Geometry check sheet. Reference: drawing and pictorial views, mm from the part's lowest x, y, z. A direction names the side the tool comes from. Give positions to 0.01 mm unless a question says otherwise; leave off trailing zeros. Write each loop counter-clockwise with the first axis right and the second up, starting at its lowest first coordinate (ties: lowest second). Pieces come first, ordered by that corner, then holes. Notation, with made-up numbers: M 8.25,35 L 43.25,35 A19 cw 43.25,55 Z; hole C 48.25,20 d1. An arc over 180 degrees is marked long. Answer as a JSON object with one key per item and string values.
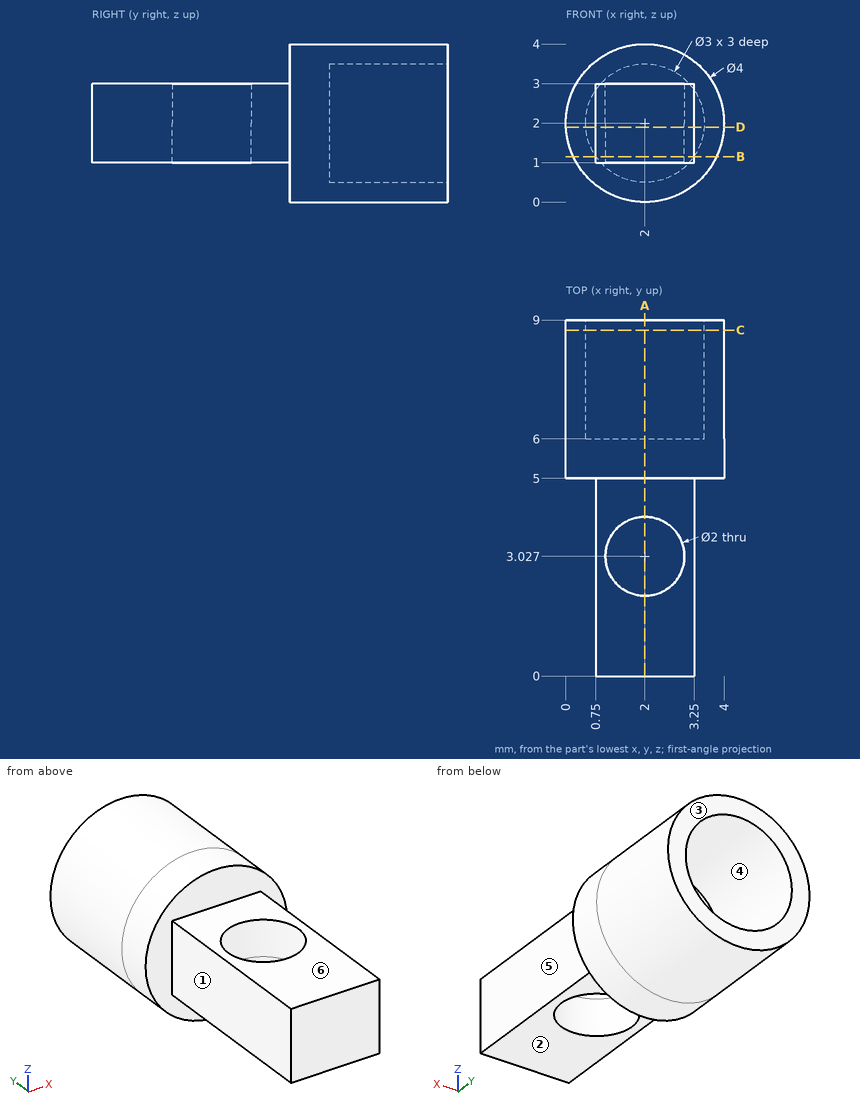
1) Section check D-D on z = 1.9. Record the boundary of the cut face in (x, y), and give its area (3 significant figures).
Completed:
{"outline": "M 0,5 L 0.75,5 L 0.75,0 L 3.25,0 L 3.25,5 L 4,5 L 4,9 L 3.5,9 L 3.5,6 L 0.5,6 L 0.5,9 L 0,9 Z; hole C 2,3.03 d2", "area": "16.4 mm2"}
2) Section check B-B on z = 1.15. Record the boundary of the cut face in (x, y).
Completed:
{"outline": "M 0.19,5 L 0.75,5 L 0.75,0 L 3.25,0 L 3.25,5 L 3.81,5 L 3.81,9 L 3.24,9 L 3.24,6 L 0.76,6 L 0.76,9 L 0.19,9 Z; hole C 2,3.03 d2"}
3) Thickness scan on L1, parallel to Y at x = 2, z = 2.6; L2, parallel to Z at x = 2, y = 6.8; L3, parallel to Y at x = 3.55, z = 1.8. Record the ranges inside material, lowest first.
Completed:
{"L1": "y = 0 to 2.03, 4.03 to 6", "L2": "z = 0 to 0.5, 3.5 to 4", "L3": "y = 5 to 9"}
4) Go/stop test with flat-tipped pins: pin 1 (1.6 mm diameter, centred on y = 2.5, z = 2, fed in from +X); pin 2 (1.2 mm diameter, centred on x = 1.5, y = 2.5, fed in from -Z); pin 3 (1 mm diameter, centred on x = 1, y = 5, fed in from -Z). Record where each tip stops, or that it passes through.
Completed:
{"pin 1": "stops at x = 3.25", "pin 2": "stops at z = 1", "pin 3": "stops at z = 0.06"}
5) Release check for a two-part mould opening along Z. For the marked faces 4, 5 and 6 record: pulls with the +Z half, pulls with the -Z half, needs draft (parallel to the pull), parting line crosses it, or undercut.
Completed:
{"face 4": "undercut", "face 5": "needs draft", "face 6": "pulls with the +Z half"}
6) Section check A-A on x = 2. Record the boundary of the cut face in (y, z).
Completed:
{"outline": "M 0,1 L 2.03,1 L 2.03,3 L 0,3 Z; M 4.03,1 L 5,1 L 5,0 L 9,0 L 9,0.5 L 6,0.5 L 6,3.5 L 9,3.5 L 9,4 L 5,4 L 5,3 L 4.03,3 Z"}
7) Section check C-C on y = 8.75. Record the boundary of the cut face in (x, z).
Completed:
{"outline": "C 2,2 d4; hole C 2,2 d3"}
8) Access from +Z, -Z, +X, -X, +Y, -Y to the whole of each face (thin tool, end or side, straight path). Record for the marked faces 1, 2 and 3.
Completed:
{"face 1": "+Z, -Z, -X, -Y", "face 2": "-Z, +X, -X, -Y", "face 3": "+Z, -Z, +X, -X, +Y"}
